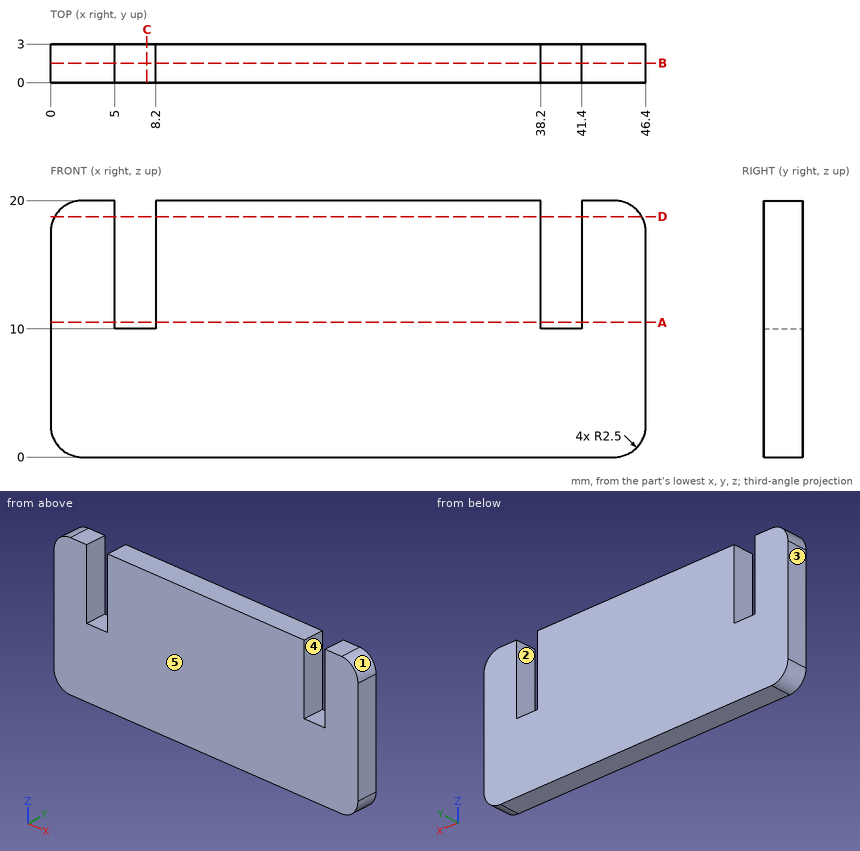
Study the drawing (mm; zero at the part's minimum x, y, z) and answer. A direction names the side the tool comes from. Round coordinates to 2 decimals unless told otherwise and drop trailing zeros. Order: outer loops, then holes, each group sorted by start corner. A loop starts at its lowest first (then second) coordinate and runs counter-clockwise, first axis right, second up. Notation, with made-up numbers: (15.5, 51.5) -> (46.5, 51.5) arc R22 ccw to (46.5, 65.5) -> close; hole circle Ø3 at (78.5, 74.5). An arc over 180 degrees is marked (long way). Answer as CSV lines item,"result". Start each with the question number.
(1) The part is cut by section B-B (y = 1.5). Determine the outline of the cut face in (x, z).
(2) A tool of negligible diameter and unlimited length cuts with its end or side. For the marked faces 4 and 5, from which of +Z, -Z, +X, -X, +Y, -Y can it reach the whole face along a straight path? Write none if from no direction.
(3) Find the intervals of material crossed by probe 1 along X at (y, z) = (0.5, 12.75); probe 2 along X at (y, z) = (0.2, 18.25); probe 3 along Z at (x, y) = (6, 2.5), in increasing order. Write a range as from..to.
(4) The part is cut by section C-C (x = 7.5). Determine the outline of the cut face in (y, z), then the cut area to 3 significant figures.
(5) The part is cut by section A-A (z = 10.5). Determine the outline of the cut face in (x, y), then the cut area to 3 significant figures.
(6) A flat-ended cylindrical pin translates along its axis: pin 1 Ø0.9 at (x, y) = (40, 1) entering from +Z. Find the tip coordinate at first contact, or state that the pin passes through.
(7) The part is cut by section D-D (z = 18.75). Determine the outline of the cut face in (x, y), then the cut area to 3 significant figures.
(8) For a pull along X with two mould halves and no side action, classify the marked faces 1, 2 and 3 as +X half, -X half, draft (parallel to the pull), parting line (faces both ways), or undercut.
Evaluation:
1,outline,"(0, 2.5) arc R2.5 ccw to (2.5, 0) -> (43.9, 0) arc R2.5 ccw to (46.4, 2.5) -> (46.4, 17.5) arc R2.5 ccw to (43.9, 20) -> (41.4, 20) -> (41.4, 10) -> (38.2, 10) -> (38.2, 20) -> (8.2, 20) -> (8.2, 10) -> (5, 10) -> (5, 20) -> (2.5, 20) arc R2.5 ccw to (0, 17.5) -> close"
2,face 4,"+Z, +Y, -Y"
2,face 5,"+Z, -Z, +X, -X, -Y"
3,probe 1,"0..5, 8.2..38.2, 41.4..46.4"
3,probe 2,"0.12..5, 8.2..38.2, 41.4..46.28"
3,probe 3,"0..10"
4,outline,"(0, 0) -> (3, 0) -> (3, 10) -> (0, 10) -> close"
4,area,"30.0 mm²"
5,outline,"(0, 0) -> (5, 0) -> (5, 3) -> (0, 3) -> close; (8.2, 0) -> (38.2, 0) -> (38.2, 3) -> (8.2, 3) -> close; (41.4, 0) -> (46.4, 0) -> (46.4, 3) -> (41.4, 3) -> close"
5,area,"120 mm²"
6,pin 1,"z = 10"
7,outline,"(0.33, 0) -> (5, 0) -> (5, 3) -> (0.33, 3) -> close; (8.2, 0) -> (38.2, 0) -> (38.2, 3) -> (8.2, 3) -> close; (41.4, 0) -> (46.07, 0) -> (46.07, 3) -> (41.4, 3) -> close"
7,area,"118 mm²"
8,face 1,"+X half"
8,face 2,"undercut"
8,face 3,"-X half"
